Autodesk Inventor part; units mm, degrees
ref_plane "YZ Plane" through (0, 0, 0) normal (1, 0, 0) x (0, 1, 0)
ref_plane "XZ Plane" through (0, 0, 0) normal (0, 1, 0) x (-1, 0, 0)
ref_plane "XY Plane" through (0, 0, 0) normal (0, 0, 1) x (1, 0, 0)
sketch "スケッチ1" plane through (0, 0, 0) normal (0, 0, 1) x (1, 0, 0)
  line L0 (0, 0) -> (15, 0)
  line L1 (15, 0) -> (15, 1.5)
  line L2 (15, 1.5) -> (0, 1.5)
  line L3 (0, 1.5) -> (0, 0)
  line L4 (0, 0) -> (0, 2.75)
  line L5 (0, 0) -> (-2, 0)
  line L6 (-2, 0) -> (0, 0)
  line L7 (-2, 0) -> (-2, 1.15)
  arc A0 (0, 2.75) -> (-2, 1.15) centre (-0.0403, 0.7504) ccw
  dimension "d0" = 1.5
  dimension "d1" = 15
  dimension "d3" = 2
  dimension "d4" = 2.75
  dimension "d5" = 1.15
  dimension "d6" = 2
revolve "回転1" add sketch "スケッチ1" angle 360 about axis through (-2, 0, 0) along (1, 0, 0)
thread "ねじ1"
sketch "スケッチ2" plane through (-2, 0, 0) normal (-1, 0, 0) x (0, 0, 1)
  circle A0 centre (0, 0) radius 1.15
  line L0 (-0.575, 0.9959) -> (0.575, 0.9959)
  line L1 (0.575, 0.9959) -> (1.15, 0)
  line L2 (1.15, 0) -> (0.575, -0.9959)
  line L3 (0.575, -0.9959) -> (-0.575, -0.9959)
  line L4 (-0.575, -0.9959) -> (-1.15, 0)
  line L5 (-1.15, 0) -> (-0.575, 0.9959)
  dimension "d10" = 1.15
  dimension "d11" = 1.9919
extrude "押し出し1" cut sketch "スケッチ2" against normal blind 1.4 contours L2 L3 L4 L5 L0 L1
fillet "フィレット1" radius 0.2 6 edges at (-0.6, 0.9959, 0) (-0.6, 0.498, 0.8625) (-0.6, 0.498, -0.8625) (-0.6, -0.498, -0.8625) (-0.6, -0.9959, 0) (-0.6, -0.498, 0.8625)
fillet "フィレット2" radius 0.1 1 edges at (0, -1.5, 0)
fillet "フィレット3" radius 0.1 1 edges at (15, -1.5, 0)
properties part number "ネジボタンM3L15" material "鋼"
The model under review builds one solid part; all positions refer to its coordinate system, in mm. A direction names the side the tool comes from. Give positions to 0.01 mm unless a question says otherwise; leave off trailing zeros. Write each loop counter-clockwise with the first axis right and the second up, starting at its lowest first coordinate (ties: lowest second). Pieces come first, ordered by that corner, then holes.
(1) The part is to be moulded in two halves that separate along Y. For faces 1 (the flat face through (0, 2, 0)), 2 (the flat face through (-1.408, 0.491, -0.867)), 3 (the cylindrical face through (7.4, -1.5, -0.07)), say which applies: released by +Y, released by -Y, zero draft, split by the parting line, or undercut.
(2) For P1, Ø2, axis at x = 10, y = -1, coming from the -Z side; P2, Ø1.5, axis at x = 7, z = -2, coming from the +Y side; P3, Ø1.3, axis at x = -1, z = 0, coming from the -Y side, all flat-tipped, find the tip position at first contact; note any pin that passes through.
(3) Consider section A-A, the plane x = 2.5. Give the boundary of the cut face in (y, z), and give its area (3 significant figures).
(4) Tool access review of faces 4 (the flat face through (-0.6, 0, 0)), 5 (the flat face through (15, 0, 0)): name each direction out of +Z, -Z, +X, -X, +Y, -Y from which nothing blocks a thin tool from reaching the whole face with its end or side.
(5) To check wall thickness, follow L1, parallel to X at y = 0.65, z = -0.1; L2, parallel to Y at x = 9.5, z = 0.55; L3, parallel to X at y = 2.35, z = -0.55. State the ranges of each line that lie inside material, in increasing order.
Returned:
1. face 1: zero draft
1. face 2: undercut
1. face 3: split by the parting line
2. P1: stops at z = -1.5
2. P2: stops at y = 0.83
2. P3: stops at y = -2.73
3. outline: circle Ø3 at (0, 0)
3. area: 7.07 mm2
4. face 4: -X
4. face 5: +Z, -Z, +X, +Y, -Y
5. L1: x = -0.6 to 15
5. L2: y = -1.4 to 1.4
5. L3: x = -1.15 to 0
